Autodesk Inventor part; units mm, degrees
ref_plane "YZ Plane" through (0, 0, 0) normal (1, 0, 0) x (0, 1, 0)
ref_plane "XZ Plane" through (0, 0, 0) normal (0, 1, 0) x (-1, 0, 0)
ref_plane "XY Plane" through (0, 0, 0) normal (0, 0, 1) x (1, 0, 0)
sketch "Skizze1" plane through (0, 0, 0) normal (0, 0, 1) x (1, 0, 0)
  line L0 (-18.1618, 0.375) -> (-21.3761, 7.875)
  line L1 (-2.9476, 7.875) -> (-6.1618, 0.375)
  line L2 (-6.1618, 0.375) -> (-18.1618, 0.375)
  line L3 (-18.1618, 0.375) -> (-31.1618, 0.375)
  line L4 (-31.1618, 0.375) -> (-31.1618, 11.375)
  line L5 (-31.1618, 11.375) -> (6.8382, 11.375)
  line L6 (6.8382, 11.375) -> (6.8382, 0.375)
  line L7 (6.8382, 0.375) -> (-6.1618, 0.375)
  line L8 (-21.5376, 7.875) -> (-2.9476, 7.875)
  point P0 (0, 0)
  point P1 (-21.1618, 7.375)
  point P2 (-3.1618, 7.375)
  dimension "d10" = 38
  dimension "d14" = 12
  dimension "d29" = 13
extrude "Extrusion1" add sketch "Skizze1" along normal blind 50 contours L3 L4 L5 L6 L7 L1 L8 L0
sketch "Skizze2" plane through (6.8382, 0.375, 0) normal (1, 0, 0) x (0, 0, -1)
  line L0 (-50, 0) -> (-50, 11)
  line L1 (0, 11) -> (-50, 11)
  point P0 (0, -0.375)
  point P1 (-25, 4.85)
  dimension "d19" = 6.15
hole "Bohrung1" at (6.8382, 5.225, 25) direction (-1, 0, 0) diameter 2.9 depth 8 tip angle 118
sketch "Skizze3" plane through (-21.3761, 7.875, 0) normal (0, -1, 0) x (1, 0, 0)
  line L0 (0, 50) -> (18.4286, 50)
  line L1 (28.2143, 0) -> (28.2143, 50)
  point P0 (21.3761, 0)
sketch "Skizze5" plane through (-31.1618, 11.375, 0) normal (0, 1, 0) x (1, 0, 0)
  line L0 (0, 0) -> (0, -50)
  line L1 (38, 0) -> (0, 0)
  circle A0 centre (19, -25) radius 7.5
  circle A1 centre (19, -25) radius 10
  point P0 (31.1618, 0)
  dimension "d39" = 19
  dimension "d40" = 25
  dimension "d41" = 15
  dimension "d42" = 20
extrude "Extrusion2" add sketch "Skizze5" along normal blind 15
ref_plane "Arbeitsebene1" through (-2.1618, 11.375, 25) normal (-1, 0, 0) x (0, -1, 0)
sketch "Skizze6" plane through (-2.1618, 11.375, 25) normal (-1, 0, 0) x (0, -1, 0)
  line L0 (-15, 10) -> (-15, -10)
  point P0 (11.375, -25)
  point P1 (-11.5, 0)
  dimension "d45" = 3.5
hole "Bohrung3" at (-2.1618, 22.875, 25) direction (-1, 0, 0) diameter 3 depth 8 tip angle 118
properties part number "7.1 Schlitten"
CAD build for the part. Positions are in the model's coordinates, mm. A direction names the side the tool comes from. Coordinates: 2 decimals unless noted, no trailing zeros. Order: outer loops, then holes, each group sorted by start corner. A loop starts at its lowest first (then second) coordinate and runs counter-clockwise, first axis right, second up. Notation, with made-up numbers: (89.5, -5.5) - (118.5, -5.5) arc R9 ccw to (118.5, 9.5) - close; hole circle Ø6 at (-15, 19.25). An arc over 180 degrees is marked (long way). Use a Markdown table: item, result. Add a question column.
(1) Which spindle directions (+Z, -Z, +X, -X, +Y, -Y) get a long thin tool onto all of the face, cutting with end or side? Do faces 4 (the face through (-12, 11.375, 25)), 5 (the face through (-4.53, 4.18, 24.65)), 6 (the face through (-3.51, 22.42, 23.57)). Say none if no direction does.
(2) Drill centre lines: line 1 along X through (y, z) = (19.25, 25); line 2 along X through (y, z) = (24.25, 20.5); line 3 along Y through (x, z) = (-20, 18) (3 decimals). Where is each one in solid material? Low to high. Write a range as [from, to].
(3) Saw through at A-A (y = 2.5). Give the cut face in (x, z).
(4) Saw through at D-D (x = 1.5). Give the cut face in (y, z) (3 decimals).
(5) Flat gauge pins, fed straight in: pin 1 (4 mm diameter, centred on y = 22.875, z = 25, fed in from +X); pin 2 (1.7 mm diameter, centred on y = 5.225, z = 25, fed in from +X); pin 3 (10 mm diameter, centred on x = -1.5, z = 39.5, fed in from +Y) (3 decimals). Where does each tip first touch, or does it go through?
(6) Saw through at B-B (z = 45). Give the cut face in (x, y) (3 decimals), then the cut area to 3 significant figures.
(7) Pull direction Z, two halves, no side cores. Call faces 1 (the face through (2.78, 5.78, 23.66)), 2 (the face through (-12.4, 8.4, 50)), 3 (the face through (-9, 26.375, 18)): +Z half, -Z half, draft (parallel to the pull), parting line (faces both ways), or undercut.
(8) Saw through at C-C (x = -9). Give the cut face in (y, z) (3 decimals).
Solved:
| question | item | result |
|---|---|---|
| 1 | face 4 | +Y |
| 1 | face 5 | +Z, -Z |
| 1 | face 6 | +X |
| 2 | line 1 | x = [-22.16, -19.66], [-4.66, -2.16] |
| 2 | line 2 | x = [-21.09, -18.16], [-6.16, -3.23] |
| 2 | line 3 | y = [0.375, 4.664], [7.875, 11.375] |
| 3 | outline | (-31.16, 0) - (-19.07, 0) - (-19.07, 50) - (-31.16, 50) - close; (-5.25, 0) - (6.84, 0) - (6.84, 50) - (-5.25, 50) - close |
| 4 | outline | (0.375, 0) - (11.375, 0) - (11.375, 50) - (0.375, 50) - close; hole circle Ø2.9 at (5.225, 25) |
| 5 | pin 1 | stops at x = -2.16 |
| 5 | pin 2 | stops at x = -1.52 |
| 5 | pin 3 | stops at y = 11.375 |
| 6 | outline | (-31.162, 0.375) - (-18.162, 0.375) - (-21.376, 7.875) - (-2.948, 7.875) - (-6.162, 0.375) - (6.838, 0.375) - (6.838, 11.375) - (-31.162, 11.375) - close |
| 6 | area | 304 mm² |
| 7 | face 1 | undercut |
| 7 | face 2 | +Z half |
| 7 | face 3 | draft |
| 8 | outline | (7.875, 0) - (11.375, 0) - (11.375, 15.513) - (26.375, 15.513) - (26.375, 18.199) - (11.375, 18.199) - (11.375, 31.801) - (26.375, 31.801) - (26.375, 34.487) - (11.375, 34.487) - (11.375, 50) - (7.875, 50) - close |
